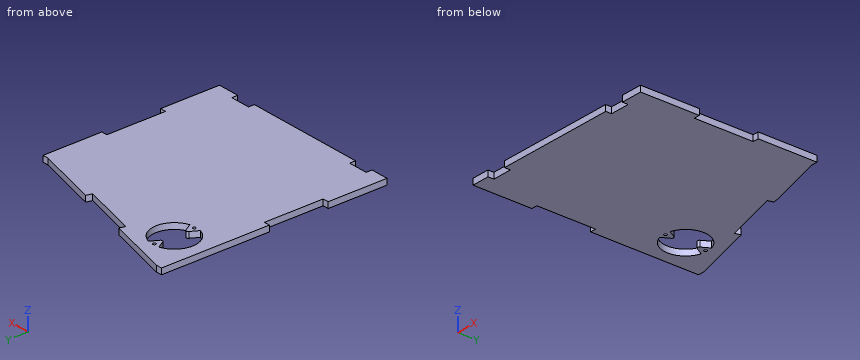
from build123d import *

# Parameters (mm, degrees)
MODEL_R             = 0.75
BOSS_EXTRUDE1_DEPTH = 3


with BuildPart() as part:
    # Model → Boss-Extrude1 (new body)
    with BuildSketch(Plane.XY):
        Polygon((403.601129512, 194.969765788), (403.601129512, 164.969765788), (406.601129512, 164.969765788), (406.601129512, 134.969765788), (395.601129512, 134.969765788), (395.601129512, 137.969765788), (385.601129512, 137.969765788), (385.601129512, 134.969765788), (324.601129512, 134.969765788), (324.601129512, 137.969765788), (314.601129512, 137.969765788), (314.601129512, 134.969765788), (305.601129512, 134.969765788), (305.601129512, 164.969765788), (308.601129512, 164.969765788), (308.601129512, 194.969765788), (305.601129512, 194.969765788), (305.601129512, 249.969765788), (308.601129512, 249.969765788), (341.595011453, 241.287165277), (340.831531555, 238.385941665), (369.843767673, 230.751142687), (370.607247571, 233.652366299), (403.601129512, 224.969765788), (406.601129512, 224.969765788), (406.601129512, 194.969765788), align=None)
        with Locations((322.652388944, 239.181914498)):
            Circle(MODEL_R, mode=Mode.SUBTRACT)
        with Locations((322.652388944, 218.781914498)):
            Circle(MODEL_R, mode=Mode.SUBTRACT)
        with BuildLine():
            Line((319.522778631, 239.551528485), (321.814644014, 235.581901198))
            ThreePointArc((321.814644014, 235.581901198), (322.680669418, 235.081901198), (323.546694821, 235.581901198))
            Line((323.546694821, 235.581901198), (325.830243575, 239.537123662))
            ThreePointArc((325.830243575, 239.537123662), (333.675600842, 228.981914498), (325.830243575, 218.426705335))
            Line((325.830243575, 218.426705335), (323.522241062, 222.353132192))
            ThreePointArc((323.522241062, 222.353132192), (322.656242047, 222.846375297), (321.794122171, 222.346382924))
            Line((321.794122171, 222.346382924), (319.522778631, 218.412300511))
            ThreePointArc((319.522778631, 218.412300511), (311.629177046, 228.981914498), (319.522778631, 239.551528485))
        make_face(mode=Mode.SUBTRACT)
    extrude(amount=BOSS_EXTRUDE1_DEPTH)


solid = part.part
The listing builds one solid part. Answer for the finished solid, in the listing's coordinates (mm). Coordinates: 2 decimals unless noted, no trailing zeros. Loops run counter-clockwise (first coordinate to the right, second up) from the corner with the lowest first, then second, coordinate; pieces in that order, holes last. Notation, with made-up numbers: M -29,58.25 L -1,58.25 A31 ccw -1,88.25 Z; hole C 26,16 d9. An arc over 180 degrees is marked long. Answer in a Markdown table with one row per item.
1) Find section C-C (z = 0.85). Count the separate pieces of the cut face and the enclosed holes in it, then the cut area to 3 significant figures.
Answers below:
| item | result |
|---|---|
| separate pieces | 1 |
| enclosed holes | 3 |
| area | 9,670 mm^2 |
2) Find the intervals of material crossed by probe 1 along Y at (x, z) = (323, 0.8); probe 2 along X at (y, z) = (221, 0.55); probe 3 along X at (y, z) = (179, 1.3), in increasing order.
Answers below:
| item | result |
|---|---|
| probe 1 | 137.97 to 218.12, 219.45 to 222.79, 235.13 to 238.52, 239.85 to 246.18 |
| probe 2 | 305.6 to 315.05, 321.02 to 324.32, 330.26 to 406.6 |
| probe 3 | 308.6 to 403.6 |
3) Find section A-A (x = 318). Determine the outline of the cut face in (y, z).
Answers below:
| item | result |
|---|---|
| outline | M 137.97,0 L 218.99,0 L 218.99,3 L 137.97,3 Z; M 238.98,0 L 247.5,0 L 247.5,3 L 238.98,3 Z |
4) Find section D-D (x = 381.5). Determine the outline of the cut face in (y, z).
Answers below:
| item | result |
|---|---|
| outline | M 134.97,0 L 230.79,0 L 230.79,3 L 134.97,3 Z |
5) Find section B-B (x = 345.5). Determine the outline of the cut face in (y, z).
Answers below:
| item | result |
|---|---|
| outline | M 134.97,0 L 237.16,0 L 237.16,3 L 134.97,3 Z |
